from build123d import *

# Parameters (mm, degrees)
BOSS_EXTRUDE1_DEPTH = 100
SKETCH2_W           = 133.34
SKETCH2_H           = 143.88
BOSS_EXTRUDE2_DEPTH = 6.35
SKETCH3_W           = 87.34
SKETCH3_H           = 56.97
BOSS_EXTRUDE3_DEPTH = 15
SKETCH4_R           = 4.5
CUT_EXTRUDE1_DEPTH  = 256.936366505
SKETCH5_W           = 40
SKETCH5_H           = 31
CUT_EXTRUDE2_DEPTH  = 251.836448109
CUT_EXTRUDE3_DEPTH  = 2.545
SKETCH7_W           = 8.71
SKETCH7_H           = 8.71
CUT_EXTRUDE4_DEPTH  = 257.878530097


with BuildPart() as part:
    # Sketch1 → Boss-Extrude1 (new body)
    with BuildSketch(Plane.XY):
        Polygon((0, 0), (0, 166.26), (-170.56, 166.26), (-170.56, 0), (-151.95, 0), (-151.95, 9.64), (-161.48, 9.64), (-161.48, 13.61), (-151.95, 13.61), (-151.95, 157.49), (-18.61, 157.49), (-18.61, 13.61), (-9.08, 13.61), (-9.08, 9.64), (-18.61, 9.64), (-18.61, 0), align=None)
    extrude(amount=BOSS_EXTRUDE1_DEPTH)

    # Sketch2 → Boss-Extrude2 (add)
    with BuildSketch(Plane(origin=(0, 0, 0), x_dir=(-1, 0, 0), z_dir=(0, 0, -1))):
        with Locations((85.28, 85.55)):
            Rectangle(SKETCH2_W, SKETCH2_H)
    extrude(amount=-BOSS_EXTRUDE2_DEPTH)

    # Sketch3 → Boss-Extrude3 (add)
    with BuildSketch(Plane.XY.offset(6.35)):
        with Locations((-108.28, 62.455)):
            Rectangle(SKETCH3_W, SKETCH3_H)
    extrude(amount=BOSS_EXTRUDE3_DEPTH)

    # Sketch4 → Cut-Extrude1 (cut, through all)
    with BuildSketch(Plane.XY.offset(6.35)):
        with Locations((-56.502483378, 39.035418079)):
            Circle(SKETCH4_R)
        with Locations((-144.227493726, 97.982911805)):
            Circle(SKETCH4_R)
    extrude(amount=-CUT_EXTRUDE1_DEPTH, mode=Mode.SUBTRACT)

    # Sketch5 → Cut-Extrude2 (cut, through all)
    with BuildSketch(Plane.XY.offset(21.35)):
        with Locations((-90.33, 57.45)):
            Rectangle(SKETCH5_W, SKETCH5_H)
    extrude(amount=-CUT_EXTRUDE2_DEPTH, mode=Mode.SUBTRACT)

    # Sketch6 → Cut-Extrude3 (cut)
    with BuildSketch(Plane.XY.offset(6.35)):
        Polygon((-77.52, 157.49), (-77.52, 135.02), (-72.88, 135.02), (-72.88, 107.08), (-98.28, 107.08), (-98.28, 135.02), (-93.64, 135.02), (-93.64, 157.49), align=None)
    extrude(amount=-CUT_EXTRUDE3_DEPTH, mode=Mode.SUBTRACT)

    # Sketch7 → Cut-Extrude4 (cut, through all)
    with BuildSketch(Plane.XY.offset(3.805)):
        with Locations((-85.575, 122.315)):
            Rectangle(SKETCH7_W, SKETCH7_H)
    extrude(amount=-CUT_EXTRUDE4_DEPTH, mode=Mode.SUBTRACT)


solid = part.part
Build history of the part. All positions in model axes, mm. A direction names the side the tool comes from. Give positions to 0.01 mm unless a question says otherwise; leave off trailing zeros. Loops run counter-clockwise (first coordinate to the right, second up) from the corner with the lowest first, then second, coordinate; pieces in that order, holes last. Notation, with made-up numbers: (61, -28.75) - (109, -28.75) arc R20 cw to (109, -17.75) - close; hole circle Ø6 at (-0.75, -30). An arc over 180 degrees is marked (long way). Write item = value, one per line. Start each with the question number.
1) Band-saw the part on A-A on y = 123. Give the cut face in (x, z) (3 decimals).
2) Drop flat-ended pins along their axis: pin 1 Ø7.5 at (x, z) = (-111.5, 13.5) entering from -Y; pin 2 Ø8 at (x, y) = (-56.5, 39.04) entering from +Z. Give the stop position or say it passes through.
3) Tool access for faces 1 (the flat face through (-84, 166.26, 49)), 2 (the flat face through (-109, 90.94, 14)), 3 (the flat face through (-18.61, 87, 53)), 4 (the flat face through (-161, 0, 49)), 5 (the flat face through (-91, 41.95, 11)): list every direction of +Z, -Z, +X, -X, +Y, -Y with a clear straight run to the whole face (end or side of a thin tool).
4) Band-saw the part on B-B on z = 27. Give the cut face in (x, y), plus the area to 3 significant figures.
5) Probe probe 1 along X at (y, z) = (109, 38.5); probe 2 along Y at (x, z) = (-154.5, 89); probe 3 along Y at (x, z) = (-37.5, 85.5). List the from-to ranges inside material, lowest first. Write a range as from..to.
6) Band-saw the part on D-D on x = -67.5. Give the cut face in (y, z), plus the area to 3 significant figures.
7) Pull direction X, two halves, no side cores. Call faces 6 (the flat face through (-84, 103, 0)), 7 (the flat face through (0, 82, 49)), 8 (the flat face through (-119, 63, 21.35)): +X half, -X half, draft (parallel to the pull), parting line (faces both ways), or undercut.
8) Band-saw the part on C-C on y = 152. Give the cut face in (x, z) (3 decimals).
Final values:
q1.outline = (-170.56, 0) - (-89.93, 0) - (-89.93, 3.805) - (-98.28, 3.805) - (-98.28, 6.35) - (-151.95, 6.35) - (-151.95, 100) - (-170.56, 100) - close; (-81.22, 0) - (0, 0) - (0, 100) - (-18.61, 100) - (-18.61, 6.35) - (-72.88, 6.35) - (-72.88, 3.805) - (-81.22, 3.805) - close
q2.pin_1 = 33.97
q2.pin_2 = through
q3.face_1 = +Z, -Z, +X, -X, +Y
q3.face_2 = +Z
q3.face_3 = +Z, -Y
q3.face_4 = +Z, -Z, +X, -X, -Y
q3.face_5 = +Z, -Z
q4.outline = (-170.56, 0) - (-151.95, 0) - (-151.95, 9.64) - (-161.48, 9.64) - (-161.48, 13.61) - (-151.95, 13.61) - (-151.95, 157.49) - (-18.61, 157.49) - (-18.61, 13.61) - (-9.08, 13.61) - (-9.08, 9.64) - (-18.61, 9.64) - (-18.61, 0) - (0, 0) - (0, 166.26) - (-170.56, 166.26) - close
q4.area = 7,280 mm²
q5.probe_1 = -170.56..-151.95, -18.61..0
q5.probe_2 = 0..9.64, 13.61..166.26
q5.probe_3 = 157.49..166.26
q6.outline = (13.61, 0) - (166.26, 0) - (166.26, 100) - (157.49, 100) - (157.49, 6.35) - (90.94, 6.35) - (90.94, 21.35) - (33.97, 21.35) - (33.97, 6.35) - (13.61, 6.35) - close
q6.area = 2,650 mm²
q7.face_6 = draft
q7.face_7 = +X half
q7.face_8 = undercut
q8.outline = (-170.56, 0) - (0, 0) - (0, 100) - (-18.61, 100) - (-18.61, 6.35) - (-77.52, 6.35) - (-77.52, 3.805) - (-93.64, 3.805) - (-93.64, 6.35) - (-151.95, 6.35) - (-151.95, 100) - (-170.56, 100) - close
